from build123d import *

# Parameters (mm, degrees)
SKETCH1_R           = 1.95
BOSS_EXTRUDE1_DEPTH = 2.5


with BuildPart() as part:
    # Sketch1 → Boss-Extrude1 (new body, symmetric)
    with BuildSketch(Plane.XY):
        with BuildLine():
            Line((133.501154847, 56.612183332), (53.501154847, 56.612183332))
            Line((53.501154847, 56.612183332), (53.501154847, 84.412183332))
            Line((53.501154847, 84.412183332), (13.501154847, 84.412183332))
            Line((13.501154847, 84.412183332), (13.501154847, 55.767785692))
            ThreePointArc((13.501154847, 55.767785692), (-49.998845153, -18.087816668), (13.501154847, -91.943419028))
            Line((13.501154847, -91.943419028), (13.501154847, -120.587816668))
            Line((13.501154847, -120.587816668), (53.501154847, -120.587816668))
            Line((53.501154847, -120.587816668), (53.501154847, -92.787816668))
            Line((53.501154847, -92.787816668), (133.501154847, -92.787816668))
            Line((133.501154847, -92.787816668), (133.501154847, -120.587816668))
            Line((133.501154847, -120.587816668), (173.501154847, -120.587816668))
            Line((173.501154847, -120.587816668), (173.501154847, -91.943419028))
            ThreePointArc((173.501154847, -91.943419028), (237.001154847, -18.087816668), (173.501154847, 55.767785692))
            Line((173.501154847, 55.767785692), (173.501154847, 84.412183332))
            Line((173.501154847, 84.412183332), (133.501154847, 84.412183332))
            Line((133.501154847, 84.412183332), (133.501154847, 56.612183332))
        make_face()
        with Locations((-41.498845153, -18.087816668)):
            Circle(SKETCH1_R, mode=Mode.SUBTRACT)
        with Locations((228.501154847, -18.087816668)):
            Circle(SKETCH1_R, mode=Mode.SUBTRACT)
        with Locations((33.501154847, 72.412183332)):
            Circle(SKETCH1_R, mode=Mode.SUBTRACT)
        with Locations((153.501154847, 72.412183332)):
            Circle(SKETCH1_R, mode=Mode.SUBTRACT)
        with Locations((33.501154847, -108.587816668)):
            Circle(SKETCH1_R, mode=Mode.SUBTRACT)
        with Locations((153.501154847, -108.587816668)):
            Circle(SKETCH1_R, mode=Mode.SUBTRACT)
    extrude(amount=BOSS_EXTRUDE1_DEPTH, both=True)


solid = part.part
Here's how the part is built. I have some questions about the finished solid (model axes, mm). Coordinates: 2 decimals unless noted, no trailing zeros. Order: outer loops, then holes, each group sorted by start corner. A loop starts at its lowest first (then second) coordinate and runs counter-clockwise, first axis right, second up. Notation, with made-up numbers: (4, -9) -> (15, -9) arc R20 ccw to (15, 19) -> close; hole circle Ø10 at (42.5, -6). An arc over 180 degrees is marked (long way). Answer in a Markdown table with one row per item.
(1) Will these pins go through, and if not, where does the flat tip stop? pin 1 Ø1.5 at (y, z) = (68, -1) entering from +X; pin 2 Ø2.5 at (y, z) = (66, 0) entering from -X; pin 3 Ø2.5 at (x, z) = (75.5, 1) entering from +Y; pin 4 Ø4.5 at (x, y) = (153.5, -108.59) entering from +Z.
Answer key:
| item | result |
|---|---|
| pin 1 | x = 173.5 |
| pin 2 | x = 13.5 |
| pin 3 | y = 56.61 |
| pin 4 | z = 2.5 |
(2) I want a section at D-D on y = -64.5. List the corners of the cut face in (x, z) for me, then the cut area to 3 significant figures.
Answer key:
| item | result |
|---|---|
| outline | (-33.83, -2.5) -> (220.83, -2.5) -> (220.83, 2.5) -> (-33.83, 2.5) -> close |
| area | 1,270 mm^2 |
(3) Please list where these lines run through material, in increasing order: probe 1 along X at (y, z) = (65, -0.35); probe 2 along Y at (x, z) = (78, 0.15); probe 3 along X at (y, z) = (20, -1.9).
Answer key:
| item | result |
|---|---|
| probe 1 | 13.5 to 53.5, 133.5 to 173.5 |
| probe 2 | -92.79 to 56.61 |
| probe 3 | -39.56 to 226.56 |
(4) I want a section at A-A on y = -101. List the corners of the cut face in (x, z) for me.
Answer key:
| item | result |
|---|---|
| outline | (13.5, -2.5) -> (53.5, -2.5) -> (53.5, 2.5) -> (13.5, 2.5) -> close; (133.5, -2.5) -> (173.5, -2.5) -> (173.5, 2.5) -> (133.5, 2.5) -> close |
(5) I want a section at C-C on x = -15. List the corners of the cut face in (y, z) for me, then the cut area to 3 significant figures.
Answer key:
| item | result |
|---|---|
| outline | (-81.36, -2.5) -> (45.19, -2.5) -> (45.19, 2.5) -> (-81.36, 2.5) -> close |
| area | 633 mm^2 |
(6) I want a section at B-B on z = -1.6. List the corners of the cut face in (x, y) for me, then the cut area to 3 significant figures.
Answer key:
| item | result |
|---|---|
| outline | (13.5, -120.59) -> (53.5, -120.59) -> (53.5, -92.79) -> (133.5, -92.79) -> (133.5, -120.59) -> (173.5, -120.59) -> (173.5, -91.94) arc R74.7 ccw to (173.5, 55.77) -> (173.5, 84.41) -> (133.5, 84.41) -> (133.5, 56.61) -> (53.5, 56.61) -> (53.5, 84.41) -> (13.5, 84.41) -> (13.5, 55.77) arc R74.7 ccw to (13.5, -91.94) -> close; hole circle Ø3.9 at (-41.5, -18.09); hole circle Ø3.9 at (33.5, -108.59); hole circle Ø3.9 at (33.5, 72.41); hole circle Ø3.9 at (153.5, -108.59); hole circle Ø3.9 at (153.5, 72.41); hole circle Ø3.9 at (228.5, -18.09) |
| area | 42,500 mm^2 |
